from build123d import *

# Parameters (mm, degrees)
F1_DEPTH = 3
F3_DEPTH = 3.001
F4_R     = 1
F5_R     = 0.2
F6_R     = 0.75
F7_DEPTH = 2.1223203436


with BuildPart() as f1:
    # F0 (on Top) → F1 (new body)
    with BuildSketch(Plane.XY):
        Polygon((17, 3), (0, 20), (0, 0), (24, 0), (24, 3.5), (22, 3.5), (22, 3), align=None)
        Polygon((12.7573593129, 3), (3, 3), (3, 12.7573593129), align=None, mode=Mode.SUBTRACT)
    extrude(amount=F1_DEPTH)

    # F2 (on face) → F3 (cut, through all)
    with BuildSketch(Plane.XY.offset(3)):
        Polygon((5.1213203436, 17.8786796564), (2.1213203436, 17.8786796564), (5.1213203436, 14.8786796564), align=None)
        Polygon((5.1213203436, 14.8786796564), (2.1213203436, 17.8786796564), (2.1213203436, 14.8786796564), align=None)
    extrude(amount=-F3_DEPTH, mode=Mode.SUBTRACT)

    # F4
    f4_edges = [f1.edges().sort_by_distance(p)[0] for p in [
        (5.12132, 14.87868, 1.5),
        (2.12132, 14.87868, 1.5),
        (3, 12.757359, 1.5),
        (17, 3, 1.5),
        (3, 3, 1.5),
        (12.757359, 3, 1.5),
        (2.12132, 17.87868, 1.5),
        (24, 0, 1.5),
        (0, 20, 1.5),
        (0, 0, 1.5),
    ]]
    fillet(f4_edges, radius=F4_R)

    # F5
    f5_edges = [f1.edges().sort_by_distance(p)[0] for p in [
        (22, 3, 1.5),
        (24, 3.5, 1.5),
        (22, 3.5, 1.5),
    ]]
    fillet(f5_edges, radius=F5_R)

    # F6 (on face) → F7 (cut, through all)
    with BuildSketch(Plane.YZ.offset(2.1213203436)):
        with Locations((16.6644660941, 1.5)):
            Circle(F6_R)
    extrude(amount=-F7_DEPTH, mode=Mode.SUBTRACT)


solid = f1.part
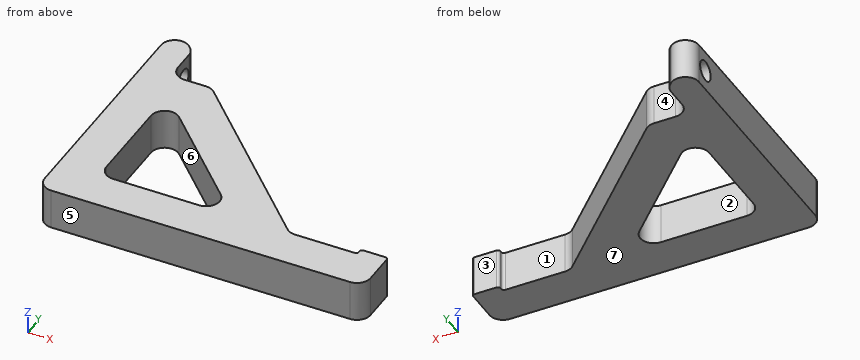
Could you check a few things on this model? Use its own coordinates, in mm. Face numbers are marked on the shaded views. A direction names the side the tool comes from. Give positions to 0.01 mm unless a question says otherwise; leave off trailing zeros. Order: outer loops, then holes, each group sorted by start corner. A loop starts at its lowest first (then second) coordinate and runs counter-clockwise, first axis right, second up. Notation, with made-up numbers: (-18.5, 36) - (13.5, 36) arc R28 ccw to (13.5, 63) - close; hole circle Ø7 at (-12.5, -26.5). An arc over 180 degrees is marked (long way). One line per item, written item: value. Start each with the question number.
1. If I drill on probe 1 along X at (y, z) = (17.5, 2.05); probe 2 along X at (y, z) = (6.5, 0.3); probe 3 along X at (y, z) = (4, 2.5), over which ranges is the centre line in solid material (lowest first)?
2. Imagine slicing it at B-B on y = 16.25. List the corners of the cut face in (x, z) for me, plus the area to 3 significant figures.
3. Imagine slicing it at C-C on x = 10.75. List the corners of the cut face in (y, z) for me.
4. For P1, Ø1.3, axis at x = 4, z = 2, coming from the +Y side; P2, Ø1.3, axis at x = 23, z = 1, coming from the +Y side; P3, Ø1.7, axis at y = 16.5, z = 2, coming from the +X side; P4, Ø0.9, axis at y = 16.66, z = 1.5, coming from the +X side (3 decimals), each with a flat end and sliding along its axis, tell me the tip position at first contact or that it passes through.
5. Imagine slicing it at D-D on x = 20.75. List the corners of the cut face in (y, z) for me.
6. Imagine slicing it at A-A on z = 1.5. Give the number of separate pieces and of enclosed holes in the cut face, plus the area to 3 significant figures.
7. For the marked faces 1, 2 and 3, which set-ups out of +Z, -Z, +X, -X, +Y, -Y let a thin tool reach every point of the face, with its end or its side?
8. Thinking about a two-plate mould opening in Y: for the marked faces 4, 5, 6 and 7, which applies, +Y half, -Y half, draft (parallel to the pull), parting line (faces both ways), or undercut?
Values:
1. probe 1: 0 to 2.12
1. probe 2: 0 to 3, 9.26 to 13.5
1. probe 3: 0 to 3, 11.34 to 16
2. outline: (0, 0) - (2.12, 0) - (2.12, 0.87) - (0, 0.87) - close; (0, 2.13) - (2.12, 2.13) - (2.12, 3) - (0, 3) - close
2. area: 3.71 mm²
3. outline: (0, 0) - (3.09, 0) - (3.09, 3) - (0, 3) - close; (5.01, 0) - (9.25, 0) - (9.25, 3) - (5.01, 3) - close
4. P1: y = 14.88
4. P2: y = 3.5
4. P3: x = 2.15
4. P4: through
5. outline: (0, 0) - (3, 0) - (3, 3) - (0, 3) - close
6. separate pieces: 2
6. enclosed holes: 1
6. area: 163 mm²
7. face 1: +Z, -Z, +Y
7. face 2: +Z, -Z
7. face 3: +Z, -Z, +X, +Y
8. face 4: +Y half
8. face 5: -Y half
8. face 6: undercut
8. face 7: draft
